```python
from build123d import *

# Parameters (mm, degrees)
SKETCH1_W          = 25.4
SKETCH1_H          = 79.375
EXTRUDE1_DEPTH     = 12.7
SKETCH2_W          = 25.4
SKETCH2_H          = 31.7754
CUT_EXTRUDE1_DEPTH = 6.477
SKETCH3_R          = 3.175
CUT_EXTRUDE2_DEPTH = 13.7
SKETCH4_R          = 5.1562
CUT_EXTRUDE3_DEPTH = 3.429


with BuildPart() as part:
    # Sketch1 → Extrude1 (new body)
    with BuildSketch(Plane.XY):
        with Locations((-17.074536082, 2.059865407)):
            Rectangle(SKETCH1_W, SKETCH1_H)
    extrude(amount=EXTRUDE1_DEPTH)

    # Sketch2 → Cut-Extrude1 (cut)
    with BuildSketch(Plane.XY.offset(12.7)):
        with Locations((-17.074536082, 2.059865407)):
            Rectangle(SKETCH2_W, SKETCH2_H)
    extrude(amount=-CUT_EXTRUDE1_DEPTH, mode=Mode.SUBTRACT)

    # Sketch3 → Cut-Extrude2 (cut, through all)
    with BuildSketch(Plane.XY.offset(12.7)):
        with BuildLine():
            ThreePointArc((-13.810636082, 10.556165407), (-17.074536082, 13.820065407), (-20.338436082, 10.556165407))
            Line((-20.338436082, 10.556165407), (-13.810636082, 10.556165407))
        make_face()
        with BuildLine():
            Line((-13.810636082, 10.556165407), (-20.338436082, 10.556165407))
            ThreePointArc((-20.338436082, 10.556165407), (-17.074536082, 7.292265407), (-13.810636082, 10.556165407))
        make_face()
        with BuildLine():
            ThreePointArc((-23.983336082, 5.323765407), (-26.291261906, 4.36779123), (-27.247236082, 2.059865407))
            Line((-27.247236082, 2.059865407), (-23.983336082, 2.059865407))
            Line((-23.983336082, 2.059865407), (-23.983336082, 5.323765407))
        make_face()
        with BuildLine():
            Line((-23.983336082, 2.059865407), (-27.247236082, 2.059865407))
            ThreePointArc((-27.247236082, 2.059865407), (-26.291261906, -0.248060416), (-23.983336082, -1.204034593))
            Line((-23.983336082, -1.204034593), (-23.983336082, 2.059865407))
        make_face()
        with BuildLine():
            Line((-23.983336082, 5.323765407), (-23.983336082, 2.059865407))
            Line((-23.983336082, 2.059865407), (-20.719436082, 2.059865407))
            ThreePointArc((-20.719436082, 2.059865407), (-21.675410259, 4.36779123), (-23.983336082, 5.323765407))
        make_face()
        with BuildLine():
            Line((-20.719436082, 2.059865407), (-23.983336082, 2.059865407))
            Line((-23.983336082, 2.059865407), (-23.983336082, -1.204034593))
            ThreePointArc((-23.983336082, -1.204034593), (-21.675410259, -0.248060416), (-20.719436082, 2.059865407))
        make_face()
        with BuildLine():
            ThreePointArc((-10.165736082, 5.323765407), (-12.473661906, 4.36779123), (-13.429636082, 2.059865407))
            Line((-13.429636082, 2.059865407), (-10.165736082, 2.059865407))
            Line((-10.165736082, 2.059865407), (-10.165736082, 5.323765407))
        make_face()
        with BuildLine():
            Line((-10.165736082, 2.059865407), (-13.429636082, 2.059865407))
            ThreePointArc((-13.429636082, 2.059865407), (-12.473661906, -0.248060416), (-10.165736082, -1.204034593))
            Line((-10.165736082, -1.204034593), (-10.165736082, 2.059865407))
        make_face()
        with BuildLine():
            Line((-10.165736082, 5.323765407), (-10.165736082, 2.059865407))
            Line((-10.165736082, 2.059865407), (-6.901836082, 2.059865407))
            ThreePointArc((-6.901836082, 2.059865407), (-7.857810259, 4.36779123), (-10.165736082, 5.323765407))
        make_face()
        with BuildLine():
            Line((-6.901836082, 2.059865407), (-10.165736082, 2.059865407))
            Line((-10.165736082, 2.059865407), (-10.165736082, -1.204034593))
            ThreePointArc((-10.165736082, -1.204034593), (-7.857810259, -0.248060416), (-6.901836082, 2.059865407))
        make_face()
        with BuildLine():
            ThreePointArc((-13.810636082, -6.436434593), (-17.074536082, -3.172534593), (-20.338436082, -6.436434593))
            Line((-20.338436082, -6.436434593), (-13.810636082, -6.436434593))
        make_face()
        with BuildLine():
            Line((-13.810636082, -6.436434593), (-20.338436082, -6.436434593))
            ThreePointArc((-20.338436082, -6.436434593), (-17.074536082, -9.700334593), (-13.810636082, -6.436434593))
        make_face()
        with Locations((-17.074536082, -24.927634593)):
            Circle(SKETCH3_R)
        with Locations((-17.074536082, 29.047365407)):
            Circle(SKETCH3_R)
    extrude(amount=-CUT_EXTRUDE2_DEPTH, mode=Mode.SUBTRACT)

    # Sketch4 → Cut-Extrude3 (cut)
    with BuildSketch(Plane.XY.offset(6.223)):
        with Locations((-17.074536082, 10.556165407)):
            Circle(SKETCH4_R)
        with Locations((-10.165736082, 2.059865407)):
            Circle(SKETCH4_R)
        with Locations((-17.074536082, -6.436434593)):
            Circle(SKETCH4_R)
        with Locations((-23.983336082, 2.059865407)):
            Circle(SKETCH4_R)
    extrude(amount=-CUT_EXTRUDE3_DEPTH, mode=Mode.SUBTRACT)


solid = part.part
```
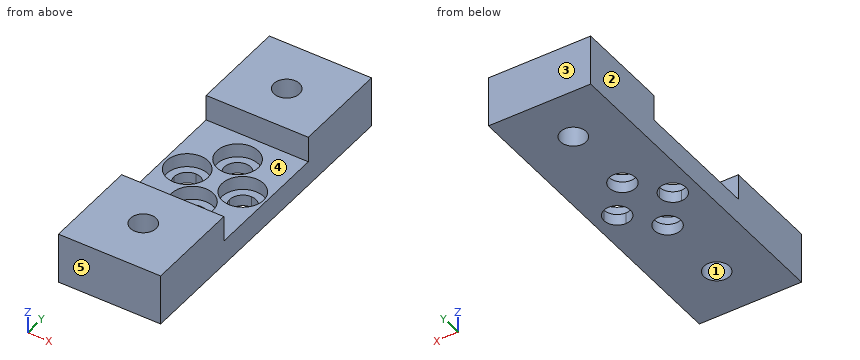
Design review of the part built by this model. Coordinates are the model's own, in mm. Face numbers are marked on the shaded views. A direction names the side the tool comes from. Round coordinates to 2 decimals unless told otherwise and drop trailing zeros. Write each loop counter-clockwise with the first axis right and the second up, starting at its lowest first coordinate (ties: lowest second). Pieces come first, ordered by that corner, then holes. Notation, with made-up numbers: (14.5, 84.25) -> (29.5, 84.25) arc R13 cw to (29.5, 95.25) -> close; hole circle Ø2 at (72, 5). An arc over 180 degrees is marked (long way). Write item = value, one per line. Start each with the question number.
1) Take a section at C-C, the plane z = 7. State the section outline as (x, y) points (3 decimals).
2) Take a section at B-B, the plane y = 4. State the section outline as (x, z) points, plus the area to 3 significant figures.
3) Take a section at A-A, the plane x = -17.5. Count the separate pieces of the cut face and the enclosed holes in it, plus the area to 3 significant figures.
4) Clearance check with flat-ended pins moving along their axes: pin 1 (13.5 mm diameter, centred on x = -23.98, y = 2.06, fed in from +Z); pin 2 (12 mm diameter, centred on x = -21, y = -14, fed in from -Z); pin 3 (9.5 mm diameter, centred on x = -17.07, y = -6.44, fed in from +Z). State where each tip first meets the part, or that it passes through.
5) Tool access review of the marked faces 4 and 5: name each direction out of +Z, -Z, +X, -X, +Y, -Y from which nothing blocks a thin tool from reaching the whole face with its end or side.
6) Wall thickness on probe 1 along Y at (x, z) = (-17.25, 8.5); probe 2 along Y at (x, z) = (-10, 3.75); probe 3 along Y at (x, z) = (-15.25, 8.25): over which ranges is each line inside the solid? List them lowest first. Write a range as from..to.
7) Mouldability with a two-part tool opening along Y and no side actions: class the marked faces 1, 2 and 3 as +Y half, -Y half, draft (parallel to the pull), parting line (faces both ways), or undercut.
8) Take a section at D-D, the plane y = -24. State the section outline as (x, z) points, plus the area to 3 significant figures.
Results list:
q1.outline = (-29.775, -37.628) -> (-4.375, -37.628) -> (-4.375, -13.828) -> (-29.775, -13.828) -> close; (-29.775, 17.948) -> (-4.375, 17.948) -> (-4.375, 41.747) -> (-29.775, 41.747) -> close; hole circle Ø6.35 at (-17.075, -24.928); hole circle Ø6.35 at (-17.075, 29.047)
q2.outline = (-29.77, 0) -> (-26.61, 0) -> (-26.61, 2.79) -> (-28.76, 2.79) -> (-28.76, 6.22) -> (-29.77, 6.22) -> close; (-21.36, 0) -> (-12.79, 0) -> (-12.79, 2.79) -> (-14.94, 2.79) -> (-14.94, 6.22) -> (-19.21, 6.22) -> (-19.21, 2.79) -> (-21.36, 2.79) -> close; (-7.54, 0) -> (-4.37, 0) -> (-4.37, 6.22) -> (-5.39, 6.22) -> (-5.39, 2.79) -> (-7.54, 2.79) -> close
q2.area = 63.2 mm²
q3.separate_pieces = 5
q3.enclosed_holes = 0
q3.area = 536 mm²
q4.pin_1 = 6.22
q4.pin_2 = 0
q4.pin_3 = 2.79
q5.face_4 = +Z, +X, -X
q5.face_5 = +Z, -Z, +X, -X, -Y
q6.probe_1 = -37.63..-28.1, -21.76..-13.83, 17.95..25.88, 32.22..41.75
q6.probe_2 = -37.63..-3.09, 7.21..41.75
q6.probe_3 = -37.63..-27.53, -22.33..-13.83, 17.95..26.45, 31.65..41.75
q7.face_1 = undercut
q7.face_2 = draft
q7.face_3 = +Y half
q8.outline = (-29.77, 0) -> (-20.11, 0) -> (-20.11, 12.7) -> (-29.77, 12.7) -> close; (-14.04, 0) -> (-4.37, 0) -> (-4.37, 12.7) -> (-14.04, 12.7) -> close
q8.area = 245 mm²
